Work out the finished part from the listing and answer in its coordinate system (mm). A direction names the side the tool comes from. Coordinates: 2 decimals unless noted, no trailing zeros. Loops run counter-clockwise (first coordinate to the right, second up) from the corner with the lowest first, then second, coordinate; pieces in that order, holes last. Notation, with made-up numbers: (62, 29.25) - (121, 29.25) arc R22 cw to (121, 68.25) - close; hole circle Ø8 at (-23.5, 45.5). An arc over 180 degrees is marked (long way). Write each question's results on one line, items separated by ' | '. Start each with the question number.
1. A cutting plane is placed at C-C on x = -5. Determine the outline of the cut face in (y, z), then the cut area to 3 significant figures.
2. Find the intervals of material crossed by line 1 along Z through (x, y) = (-4, 3.5); line 2 along X through (y, z) = (0, 7.25); line 3 along Y through (x, z) = (-3.25, 3), in increasing order. Write a range as [from, to].
3. A cutting plane is placed at A-A on x = 0. Determine the outline of the cut face in (y, z), then the cut area to 3 significant figures.
4. Which of the six approach directions +Z, -Z, +X, -X, +Y, -Y give full straight-line access (tool end or side, diameter ignored) to faces 1 (the cylindrical face through (0, 2.6, 6.4)), 2 (the flat face through (3, -4, 2)), 3 (the flat face through (2, 1, 0))?
5. A cutting plane is placed at B-B on y = 0. Determine the outline of the cut face in (x, z).
6. Determine the mould class of faces 4 (the cylindrical face through (-6, 0, 12)), 5 (the flat face through (3, 0, 13)), 6 (the flat face through (1.6, 0, 6)), 7 (the cylindrical face through (0, -2.6, 6.4)) for opening direction X: released by +X, released by -X, zero draft, split by the parting line, or undercut.
7. Each of these flat-tipped pins is pushed along its axis until it touches: P1, Ø0.6, axis at x = 0, z = 7.5, coming from the +Y side; P2, Ø3, axis at x = -4.5, z = 5, coming from the -Y side; P3, Ø1.5, axis at y = 3.5, z = 7.5, coming from the -X side. Where does it stop, or does it pass through?
from build123d import *

# Parameters (mm, degrees)
F2_DEPTH        = 13
F1_R            = 6
F3_DEPTH        = 2
F4_DEPTH        = 13
F4_COPIES_COUNT = 16


# Not quite as in the source:
# - a pattern or mirror of a feature is missing from the dataset's text; its kind, count and spacing are read off the source's solid


with BuildPart() as f2:
    # F1 (on Top) → F2 (new body)
    with BuildSketch(Plane.XY):
        with BuildLine():
            ThreePointArc((-0.7033229276, -3.9389354049), (-0.4774392089, -3.9726473625), (-0.25, -3.9934164903))
            Line((-0.25, -3.9934164903), (0.25, -3.9934164903))
            Line((0.25, -3.9934164903), (0.7033229276, -3.9389354049))
            ThreePointArc((0.7033229276, -3.9389354049), (0, 4.0012342177), (-0.7033229276, -3.9389354049))
        make_face()
        with BuildLine():
            ThreePointArc((1.6, 2.0493901532), (2.3366642891, 1.1401754251), (2.6, 0))
            ThreePointArc((2.6, 0), (2.3366642891, -1.1401754251), (1.6, -2.0493901532))
            ThreePointArc((1.6, -2.0493901532), (0, -2.6), (-1.6, -2.0493901532))
            ThreePointArc((-1.6, -2.0493901532), (-2.6, 0), (-1.6, 2.0493901532))
            ThreePointArc((-1.6, 2.0493901532), (0, 2.6), (1.6, 2.0493901532))
        make_face(mode=Mode.SUBTRACT)
        with BuildLine():
            ThreePointArc((1.6, -2.0493901532), (2.3366642891, -1.1401754251), (2.6, 0))
            ThreePointArc((2.6, 0), (2.3366642891, 1.1401754251), (1.6, 2.0493901532))
            Line((1.6, 2.0493901532), (1.6, -2.0493901532))
        make_face()
        with BuildLine():
            Line((-1.6, -2.0493901532), (-1.6, 2.0493901532))
            ThreePointArc((-1.6, 2.0493901532), (-2.6, 0), (-1.6, -2.0493901532))
        make_face()
    extrude(amount=F2_DEPTH)

    # F1 (on Top) → F3 (join)
    with BuildSketch(Plane.XY):
        Circle(F1_R)
        with BuildLine():
            ThreePointArc((-0.25, -4.4803719605), (-0.3782937101, -4.1272943414), (-0.7033229276, -3.9389354049))
            ThreePointArc((-0.7033229276, -3.9389354049), (0, 4.0012342177), (0.7033229276, -3.9389354049))
            ThreePointArc((0.7033229276, -3.9389354049), (0.3782937101, -4.1272943414), (0.25, -4.4803719605))
            Line((0.25, -4.4803719605), (0.25, -4.7434164903))
            Line((0.25, -4.7434164903), (-0.25, -4.7434164903))
            Line((-0.25, -4.7434164903), (-0.25, -4.4803719605))
        make_face(mode=Mode.SUBTRACT)
    f3 = extrude(amount=F3_DEPTH)

    # F3_copies: F3 across plane
    add(f3.mirror(Plane.XY.offset(6.5)))

    # F1 (on Top) → F4 (join)
    with BuildSketch(Plane.XY):
        with BuildLine():
            Line((0.25, -3.9934164903), (-0.25, -3.9934164903))
            ThreePointArc((-0.25, -3.9934164903), (-0.4774392089, -3.9726473625), (-0.7033229276, -3.9389354049))
            ThreePointArc((-0.7033229276, -3.9389354049), (-0.3782937101, -4.1272943414), (-0.25, -4.4803719605))
            Line((-0.25, -4.4803719605), (-0.25, -4.7434164903))
            Line((-0.25, -4.7434164903), (0.25, -4.7434164903))
            Line((0.25, -4.7434164903), (0.25, -4.4803719605))
            ThreePointArc((0.25, -4.4803719605), (0.3782937101, -4.1272943414), (0.7033229276, -3.9389354049))
            Line((0.7033229276, -3.9389354049), (0.25, -3.9934164903))
        make_face()
    f4 = extrude(amount=F4_DEPTH)

    # F4_copies: F4 ×16 about axis
    f4_copies_axis = Axis((0, 0, 0), (0, 0, 1))
    for i in range(1, F4_COPIES_COUNT):
        add(f4.rotate(f4_copies_axis, i * 360 / F4_COPIES_COUNT))


solid = f2.part
Values:
1) outline: (-3.32, 0) - (3.32, 0) - (3.32, 2) - (-3.32, 2) - close; (-3.32, 11) - (3.32, 11) - (3.32, 13) - (-3.32, 13) - close | area: 26.5 mm^2
2) line 1: [0, 2], [11, 13] | line 2: [-4.74, -1.6], [1.6, 4.74] | line 3: [-3.46, -2.86], [-2.34, 2.34], [2.86, 3.46]
3) outline: (-6, 0) - (-2.6, 0) - (-2.6, 13) - (-6, 13) - (-6, 11) - (-4.74, 11) - (-4.74, 2) - (-6, 2) - close; (2.6, 0) - (6, 0) - (6, 2) - (4.74, 2) - (4.74, 11) - (6, 11) - (6, 13) - (2.6, 13) - close | area: 65.8 mm^2
4) face 1: +Z, -Z | face 2: none | face 3: -Z, +X, -X, +Y, -Y
5) outline: (-6, 0) - (-1.6, 0) - (-1.6, 13) - (-6, 13) - (-6, 11) - (-4.74, 11) - (-4.74, 2) - (-6, 2) - close; (1.6, 0) - (6, 0) - (6, 2) - (4.74, 2) - (4.74, 11) - (6, 11) - (6, 13) - (1.6, 13) - close
6) face 4: split by the parting line | face 5: zero draft | face 6: undercut | face 7: undercut
7) P1: y = 4.74 | P2: y = -3.53 | P3: x = -3.53
